Check sheet for the modelled part. Datum: model origin and axes. Units: mm. A direction names the side the tool comes from. Give positions to 0.01 mm unless a question says otherwise; leave off trailing zeros. Write each loop counter-clockwise with the first axis right and the second up, starting at its lowest first coordinate (ties: lowest second). Pieces come first, ordered by that corner, then holes.
from build123d import *

# Parameters (mm, degrees)
F1_DEPTH = 40
F2_R     = 5


with BuildPart() as f1:
    # F0 (on Front) → F1 (new body, symmetric)
    with BuildSketch(Plane.XZ):
        with BuildLine():
            Line((0, 0), (-75, 0))
            ThreePointArc((-75, 0), (-93.22257, 7.88457), (-99.95097, 26.564963))
            Line((-99.95097, 26.564963), (-99.990197, 126.564956))
            ThreePointArc((-99.990197, 126.564956), (-107.315993, 144.236285), (-124.990195, 151.555149))
            Line((-124.990195, 151.555149), (-145, 151.555149))
            Line((-145, 151.555149), (-145, -23.444851))
            ThreePointArc((-145, -23.444851), (-137.67767, -41.122521), (-120, -48.444851))
            Line((-120, -48.444851), (120, -48.444851))
            ThreePointArc((120, -48.444851), (137.67767, -41.122521), (145, -23.444851))
            Line((145, -23.444851), (145, 151.555149))
            Line((145, 151.555149), (124.990195, 151.555149))
            ThreePointArc((124.990195, 151.555149), (107.315993, 144.236285), (99.990197, 126.564956))
            Line((99.990197, 126.564956), (99.95097, 26.564963))
            ThreePointArc((99.95097, 26.564963), (93.22257, 7.88457), (75, 0))
            Line((75, 0), (0, 0))
        make_face()
        with BuildLine():
            Line((-84.95097, -10), (0, -10))
            Line((0, -10), (81.913937, -10))
            ThreePointArc((81.913937, -10), (99.591607, -2.67767), (106.913937, 15))
            Line((106.913937, 15), (106.913937, 116.555149))
            ThreePointArc((106.913937, 116.555149), (114.236268, 134.232818), (131.913937, 141.555149))
            Line((131.913937, 141.555149), (135, 141.555149))
            Line((135, 141.555149), (135, -13.444851))
            ThreePointArc((135, -13.444851), (127.67767, -31.122521), (110, -38.444851))
            Line((110, -38.444851), (-110, -38.444851))
            ThreePointArc((-110, -38.444851), (-127.67767, -31.122521), (-135, -13.444851))
            Line((-135, -13.444851), (-135, 141.555149))
            Line((-135, 141.555149), (-134.95097, 141.555149))
            ThreePointArc((-134.95097, 141.555149), (-117.2733, 134.232818), (-109.95097, 116.555149))
            Line((-109.95097, 116.555149), (-109.95097, 15))
            ThreePointArc((-109.95097, 15), (-102.628639, -2.67767), (-84.95097, -10))
        make_face(mode=Mode.SUBTRACT)
    extrude(amount=F1_DEPTH, both=True)

    # F2
    f2_edges = [f1.edges().sort_by_distance(p)[0] for p in [
        (-145, 0, 151.555149),
        (145, 0, 151.555149),
    ]]
    fillet(f2_edges, radius=F2_R)


solid = f1.part
1) Access from +Z, -Z, +X, -X, +Y, -Y to the whole of each face (thin tool, end or side, straight path). Record for faces 1 (the cylindrical face through (-127.5, -0.6, -31.3)), 2 (the flat face through (1, -1, 0)), 3 (the cylindrical face through (137.5, -0.6, -41.3)).
2) Scan lines: L1, parallel to X at y = -33.5, z = 50; L2, parallel to Z at x = -66, y = 24.5; L3, parallel to X at y = 23, z = 131. Record each from-to range of solid material in increasing order.
3) Gauge pin test, flat ends, axial feed: pin 1 (5 mm diameter, centred on x = -69, y = 13.5, fed in from +Z); pin 2 (3.5 mm diameter, centred on x = 133, y = 0.5, fed in from -Z). Record the tip position at first contact, or that the pin passes through.
4) Draft check along X on faces 4 (the flat face through (-1, -40, -7)), 5 (the cylindrical face through (-137.9, -0.6, -40.9)), 6 (the flat face through (-109.951, -1, 66)). Enter one of: +X half, -X half, draft (parallel to the pull), parting line (faces both ways), or undercut.
5) Sectioned sample at C-C on z = 135.5. Record the boundary of the cut face in (x, y), then the cut area to 3 significant figures.
6) Sectioned sample at D-D on z = 23.5. Record the boundary of the cut face in (x, y).
7) Sectioned sample at B-B on x = -54.5. Record the boundary of the cut face in (y, z).
Answers below:
1. face 1: +Y, -Y
1. face 2: +Z, +Y, -Y
1. face 3: -Z, +X, +Y, -Y
2. L1: x = -145 to -135, -109.95 to -99.96, 99.96 to 106.91, 135 to 145
2. L2: z = -48.44 to -38.44, -10 to 0
2. L3: x = -145 to -135, -114.55 to -100.39, 100.39 to 111.51, 135 to 145
3. pin 1: stops at z = 0
3. pin 2: stops at z = -45.77
4. face 4: draft
4. face 5: -X half
4. face 6: undercut
5. outline: (-145, -40) - (-135, -40) - (-135, 40) - (-145, 40) - close; (-118.64, -40) - (-101.65, -40) - (-101.65, 40) - (-118.64, 40) - close; (101.65, -40) - (115.6, -40) - (115.6, 40) - (101.65, 40) - close; (135, -40) - (145, -40) - (145, 40) - (135, 40) - close
5. area: 4,080 mm2
6. outline: (-145, -40) - (-135, -40) - (-135, 40) - (-145, 40) - close; (-109.95, -40) - (-99.95, -40) - (-99.95, 40) - (-109.95, 40) - close; (99.95, -40) - (106.91, -40) - (106.91, 40) - (99.95, 40) - close; (135, -40) - (145, -40) - (145, 40) - (135, 40) - close
7. outline: (-40, -48.44) - (40, -48.44) - (40, -38.44) - (-40, -38.44) - close; (-40, -10) - (40, -10) - (40, 0) - (-40, 0) - close
